from build123d import *

# Parameters (mm, degrees)
SKETCH010_R          = 4.679612
POCKET005_DEPTH      = 10.301
SKETCH011_W          = 1.2
SKETCH011_H          = 6
POCKET006_DEPTH      = 2.376
POCKET006_DEPTH_BACK = 2.376


with BuildPart() as part:
    # Sketch009 → Revolution (revolve)
    with BuildSketch(Plane.XZ):
        with BuildLine():
            Line((1.4224, 0.5), (1.4224, -4.178777))
            Line((1.4224, -4.178777), (0, -5))
            Line((0, -5), (0, -11.1))
            Line((0, -11.1), (1.35, -11.1))
            Line((1.35, -11.1), (1.6, -9.7))
            Line((1.6, -9.7), (1.6, -8.3))
            Line((1.6, -8.3), (1.4, -8.3))
            Line((1.4, -8.3), (1.4, -6.8))
            Line((1.4, -6.8), (4, -6.8))
            Line((4, -6.8), (4, -0.8))
            Line((4, -0.8), (2, -0.8))
            Line((2, -0.8), (2, 0))
            Line((2, 0), (2.35, 0))
            ThreePointArc((2.35, 0), (1.949288, 0.36704), (1.4224, 0.5))
        make_face()
    revolve(axis=Axis((0, 0, 0), (0, 0, 1)))

    # Sketch010 (on Face10 of Revolution) → Pocket005 (cut, through all)
    with BuildSketch(Plane(origin=(0, 0, -0.8), x_dir=(-1, 0, 0), z_dir=(0, 0, 1))):
        Circle(SKETCH010_R)
        Polygon((0, 2.742414), (-2.375, 1.371207), (-2.375, -1.371207), (0, -2.742414), (2.375, -1.371207), (2.375, 1.371207), align=None, mode=Mode.SUBTRACT)
    extrude(amount=-POCKET005_DEPTH, mode=Mode.SUBTRACT)

    # Sketch011 → Pocket006 (cut, two sides)
    with BuildSketch(Plane.YZ) as pocket006_sk:
        with Locations((0, -8.5)):
            Rectangle(SKETCH011_W, SKETCH011_H)
    extrude(amount=-POCKET006_DEPTH, mode=Mode.SUBTRACT)
    extrude(pocket006_sk.sketch, amount=POCKET006_DEPTH_BACK, mode=Mode.SUBTRACT)


with BuildPart() as part_1:
    # Body002 placement: moved
    add(part.part.moved(Location((-31.755, 0, 0.4))))


with BuildPart() as part_2:
    # Clone placement: moved
    add(part_1.part.moved(Location((31.755, 0, -0.4))))


with BuildPart() as part_3:
    # Body003 placement: moved
    add(part_2.part.moved(Location((31.755, 0, 0.4))))


solid = part_3.part
Source: CAD feature listing. Evaluate the final solid. Frame: model axes, mm. A direction names the side the tool comes from. Round coordinates to 2 decimals unless told otherwise and drop trailing zeros. Loops run counter-clockwise (first coordinate to the right, second up) from the corner with the lowest first, then second, coordinate; pieces in that order, holes last. Notation, with made-up numbers: M 44,37 L 76,37 A23 cw 76,76 Z; hole C -29,44.25 d7. An arc over 180 degrees is marked long. Return JSON: item names as keys, results as strings. Group by question number.
1. Reachability of faces 1 (the face through (31.97, 0.07, -4.47)), 2 (the face through (31.8, 1.4, -7.1)), 3 (the face through (31.7, -1.6, -8.6)), 4 (the face through (31.8, 1.6, -8.6)), 5 (the face through (32, -0.6, -7)) from +Z, -Z, +X, -X, +Y, -Y: full face, straight path, thin tool, end or side. Return the list, or none.
2. Section query B-B on z = -8.5. Output: boundary loops of the cut face in (x, y) (3 decimals).
3. Material intervals for line 1 along X through (y, z) = (0.45, -2.5); line 2 along Y through (x, z) = (30.7, -7); line 3 along Y through (x, z) = (32, -6.5), sorted ascending. Write a range as from..to.
4. Pin query (flat end, axial travel): pin 1 (0.5 mm diameter, centred on x = 32, y = 1, fed in from +Z); pin 2 (1.5 mm diameter, centred on y = -0.5, z = -6.5, fed in from -X); pin 3 (1.5 mm diameter, centred on x = 30, z = -4.5, fed in from -Y); pin 4 (1 mm diameter, centred on x = 31, z = -8.5, fed in from +Y). Return the tip coordinate at first contact, or that it passes through.
5. Mould query, pull axis Y, two halves, no side actions, for faces 6 (the face through (32, 0.6, -7)), 7 (the face through (30.334, 0.063, -1.472)), 8 (the face through (29.38, 0, -3)), 9 (the face through (32.959, 2.047, -3.358)). Classes: released by +Y, released by -Y, zero draft, split by the parting line, or undercut.
6. Section query A-A on z = -5.5. Output: boundary loops of the cut face in (x, y) (3 decimals).
Checks:
{
 "1": {"face 1": "+Z", "face 2": "+Y", "face 3": "-Z, -Y", "face 4": "-Z, +Y", "face 5": "-Z, +X, -X"},
 "2": {"outline": "M 30.272,-0.6 A1.6 ccw 33.238,-0.6 Z; M 30.272,0.6 L 33.238,0.6 A1.6 ccw Z"},
 "3": {"line 1": "x = 29.38..30.41, 33.1..34.13", "line 2": "y = -0.92..-0.6, 0.6..0.92", "line 3": "y = -1.38..-0.6, 0.6..1.38"},
 "4": {"pin 1": "stops at z = -3.86", "pin 2": "stops at x = 29.38", "pin 3": "stops at y = -2.16", "pin 4": "stops at y = 1.58"},
 "5": {"face 6": "undercut", "face 7": "undercut", "face 8": "zero draft", "face 9": "released by +Y"},
 "6": {"outline": "M 29.38,-1.371 L 31.755,-2.742 L 34.13,-1.371 L 34.13,-0.6 L 29.38,-0.6 Z; M 29.38,0.6 L 34.13,0.6 L 34.13,1.371 L 31.755,2.742 L 29.38,1.371 Z"}
}
